Source: CAD feature listing. Evaluate the final solid. Frame: model axes, mm. Face numbers are marked on the shaded views. A direction names the side the tool comes from. Round coordinates to 2 decimals unless told otherwise and drop trailing zeros. Write each loop counter-clockwise with the first axis right and the second up, starting at its lowest first coordinate (ties: lowest second). Pieces come first, ordered by that corner, then holes. Notation, with made-up numbers: M 10,-1.75 L 16,-1.75 A27 ccw 16,26.25 Z; hole C 40.25,26.5 d11. An arc over 180 degrees is marked long. Use a Markdown table: item, result.
```python
from build123d import *

# Parameters (mm, degrees)
SKETCH2_R           = 1.75
BOSS_EXTRUDE1_DEPTH = 2.875
FILLET1_R           = 1.5875


with BuildPart() as part:
    # Sketch2 → Boss-Extrude1 (new body)
    with BuildSketch(Plane(origin=(0, 0, 0), x_dir=(0, 0, -1), z_dir=(1, 0, 0))):
        with BuildLine():
            Line((13.247387042, 2), (2.236067977, 2))
            ThreePointArc((2.236067977, 2), (-3, 0), (2.236067977, -2))
            Line((2.236067977, -2), (12.13290764, -2))
            Line((12.13290764, -2), (20.13290764, -6.833106971))
            Line((20.13290764, -6.833106971), (24.896839663, -6.833106971))
            ThreePointArc((24.896839663, -6.833106971), (30.13290764, -4.833106971), (24.896839663, -2.833106971))
            Line((24.896839663, -2.833106971), (21.247387042, -2.833106971))
            Line((21.247387042, -2.833106971), (13.247387042, 2))
        make_face()
        Circle(SKETCH2_R, mode=Mode.SUBTRACT)
        with Locations((27.13290764, -4.833106971)):
            Circle(SKETCH2_R, mode=Mode.SUBTRACT)
    extrude(amount=BOSS_EXTRUDE1_DEPTH)

    # Fillet1
    fillet1_edges = [part.edges().sort_by_distance(p)[0] for p in [
        (1.4375, -6.833106971, -24.896839663),
        (1.4375, -2, -12.13290764),
        (1.4375, -2, -2.236067977),
        (1.4375, 2, -2.236067977),
        (1.4375, -2.833106971, -21.247387042),
        (1.4375, -2.833106971, -24.896839663),
    ]]
    fillet(fillet1_edges, radius=FILLET1_R)


solid = part.part
```
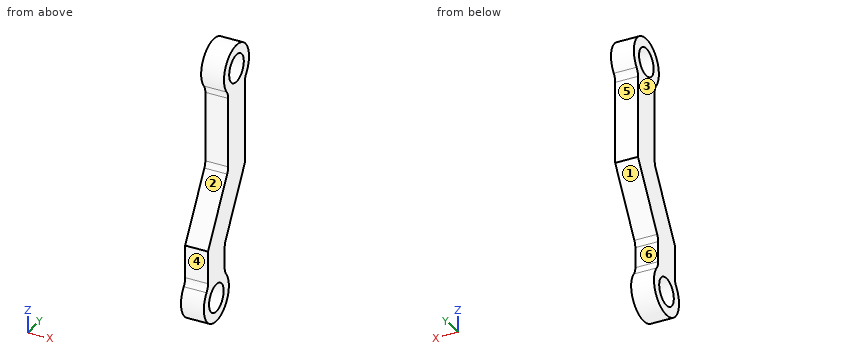
Q1. Mould query, pull axis Z, two halves, no side actions, for the marked faces 5 and 6. Classes: +Z half, -Z half, draft (parallel to the pull), parting line (faces both ways), or undercut.
Results are:
| item | result |
|---|---|
| face 5 | draft |
| face 6 | undercut |
Q2. Line query: L1, parallel to Y at x = 0.7, z = 0; L2, parallel to Z at x = 1.5, y = -2.5; L3, parallel to Y at x = 2, z = -9. Output: solid intervals per line, ascending.
Results are:
| item | result |
|---|---|
| L1 | -3 to -1.75, 1.75 to 3 |
| L2 | -29.02 to -25.25, -20.7 to -12.96, -1.66 to 1.66 |
| L3 | -2 to 2 |
Q3. Section D-D on z = -6. Return loops of the section in (x, y) (3 decimals), plus the area to 3 significant figures.
Results are:
| item | result |
|---|---|
| outline | M 0,-2 L 2.875,-2 L 2.875,2 L 0,2 Z |
| area | 11.5 mm^2 |
Q4. Reachability of the marked faces 1, 2, 3 and 4 from +Z, -Z, +X, -X, +Y, -Y: full face, straight path, thin tool, end or side. Return the list, or none.
Results are:
| item | result |
|---|---|
| face 1 | +X, -X, +Y |
| face 2 | +X, -X, -Y |
| face 3 | +Z, -Z, -X, +Y, -Y |
| face 4 | +Z, +X, -X, -Y |
Q5. First-contact query: pin 1 Ø3 at (y, z) = (0, 0) entering from +X; pin 2 Ø1.5 at (x, z) = (1, -17.5) entering from +Y; pin 3 Ø1.4 at (x, z) = (1.5, -9) entering from +Y; pin 4 Ø0.9 at (x, z) = (1.5, -22.5) entering from -Y. Flat tips, straight axial feed; report the tip coordinate or a pass-through.
Results are:
| item | result |
|---|---|
| pin 1 | through |
| pin 2 | y = -0.12 |
| pin 3 | y = 2 |
| pin 4 | y = -6.83 |
Q6. Section A-A on z = 0. Return loops of the section in (x, y) (3 decimals), plus the area to 3 significant figures.
Results are:
| item | result |
|---|---|
| outline | M 0,-3 L 2.875,-3 L 2.875,-1.75 L 0,-1.75 Z; M 0,1.75 L 2.875,1.75 L 2.875,3 L 0,3 Z |
| area | 7.19 mm^2 |
Q7. Section C-C on x = 1.35. Give the number of separate pieces and of enclosed holes in the cut face, plus the area to 3 significant figures.
Results are:
| item | result |
|---|---|
| separate pieces | 1 |
| enclosed holes | 2 |
| area | 129 mm^2 |
Q8. Section B-B on y = 0.5. Return loops of the section in (x, z) (3 decimals), plus the area to 3 significant figures.
Results are:
| item | result |
|---|---|
| outline | M 0,-15.73 L 2.875,-15.73 L 2.875,-1.677 L 0,-1.677 Z; M 0,1.677 L 2.875,1.677 L 2.875,2.958 L 0,2.958 Z |
| area | 44.1 mm^2 |
